Check sheet for the modelled part. Datum: model origin and axes. Units: mm. Face numbers are marked on the shaded views. A direction names the side the tool comes from. Give positions to 0.01 mm unless a question says otherwise; leave off trailing zeros. Write each loop counter-clockwise with the first axis right and the second up, starting at its lowest first coordinate (ties: lowest second). Pieces come first, ordered by that corner, then holes.
from build123d import *

# Parameters (mm, degrees)
F0_R     = 20
F0_R_2   = 12.5
F1_DEPTH = 30
F2_R     = 55
F2_R_2   = 20
F3_DEPTH = 25
F4_R     = 12.5
F5_DEPTH = 25


with BuildPart() as f1:
    # F0 (on Right) → F1 (new body)
    with BuildSketch(Plane.YZ):
        with BuildLine():
            ThreePointArc((22, -76.9155380921), (63.8748776907, -48.1663783152), (80, 0))
            ThreePointArc((80, 0), (63.8748776907, 48.1663783152), (22, 76.9155380921))
            ThreePointArc((22, 76.9155380921), (-80, 0), (22, -76.9155380921))
        make_face()
        Circle(F0_R, mode=Mode.SUBTRACT)
        with BuildLine():
            ThreePointArc((22, 76.9155380921), (63.8748776907, 48.1663783152), (80, 0))
            ThreePointArc((80, 0), (63.8748776907, -48.1663783152), (22, -76.9155380921))
            Line((22, -76.9155380921), (206.875, -24.0361056538))
            ThreePointArc((206.875, -24.0361056538), (175, 0), (206.875, 24.0361056538))
            Line((206.875, 24.0361056538), (22, 76.9155380921))
        make_face()
        with BuildLine():
            ThreePointArc((225, 0), (219.9608992783, 15.0519932235), (206.875, 24.0361056538))
            ThreePointArc((206.875, 24.0361056538), (175, 0), (206.875, -24.0361056538))
            ThreePointArc((206.875, -24.0361056538), (219.9608992783, -15.0519932235), (225, 0))
        make_face()
        with Locations((200, 0)):
            Circle(F0_R_2, mode=Mode.SUBTRACT)
    extrude(amount=F1_DEPTH)

    # F2 (on face) → F3 (join)
    with BuildSketch(Plane.YZ.offset(30)):
        Circle(F2_R)
        Circle(F2_R_2, mode=Mode.SUBTRACT)
    extrude(amount=F3_DEPTH)

    # F4 (on face) → F5 (join)
    with BuildSketch(Plane.YZ.offset(30)):
        with BuildLine():
            ThreePointArc((206.875, -24.0361056538), (219.9608992783, -15.0519932235), (225, 0))
            ThreePointArc((225, 0), (219.9608992783, 15.0519932235), (206.875, 24.0361056538))
            ThreePointArc((206.875, 24.0361056538), (175, 0), (206.875, -24.0361056538))
        make_face()
        with Locations((200, 0)):
            Circle(F4_R, mode=Mode.SUBTRACT)
    extrude(amount=F5_DEPTH)


solid = f1.part
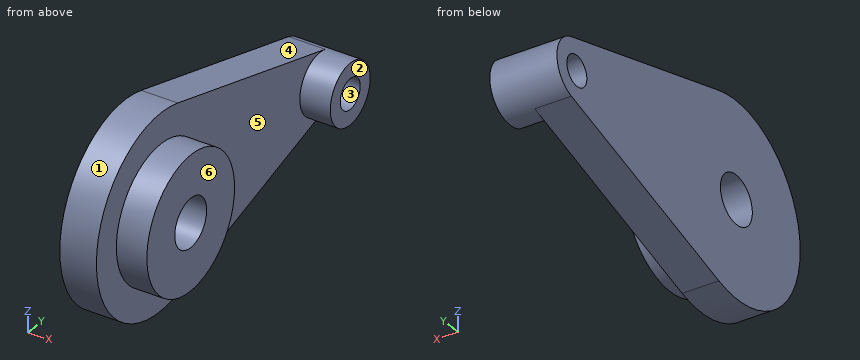
1) Draft check along Z on the marked faces 1, 2, 3 and 4. Enter one of: +Z half, -Z half, draft (parallel to the pull), parting line (faces both ways), or undercut.
2) Gauge pin test, flat ends, axial feed: pin 1 (5 mm diameter, centred on x = 12.5, z = 33.5, fed in from -Y); pin 2 (1 mm diameter, centred on x = 35, y = 47, fed in from -Z); pin 3 (6 mm diameter, centred on x = 42, y = -27.5, fed in from +Z); pin 4 (1.5 mm diameter, centred on y = 78.5, z = -31, fed in from -X). Record the tip position at first contact, or that the pin passes through.
3) Sectioned sample at C-C on x = 12. Record the boundary of the cut face in (y, z) (3 decimals), then the cut area to 3 significant figures.
4) Sectioned sample at A-A on z = 0. Record the boundary of the cut face in (x, y).
5) Scan lines: L1, parallel to Z at x = 32.5, y = 0; L2, parallel to Z at x = 20, y = 0; L3, parallel to X at y = -39, z = -55. Record each from-to range of solid material in increasing order.
6) Sectioned sample at D-D on x = 51. Record the boundary of the cut face in (y, z) (3 decimals), then the cut area to 3 significant figures.
7) Access from +Z, -Z, +X, -X, +Y, -Y to the whole of each face (thin tool, end or side, straight path). Record for the marked faces 5 and 6.
8) Sectioned sample at B-B on y = 0. Record the boundary of the cut face in (x, z).
Answers below:
1. face 1: parting line
1. face 2: draft
1. face 3: undercut
1. face 4: +Z half
2. pin 1: stops at y = -73.75
2. pin 2: stops at z = -29.37
2. pin 3: stops at z = 49.24
2. pin 4: stops at x = 0
3. outline: (22, -76.916) - (206.875, -24.036) arc R25 ccw to (206.875, 24.036) - (22, 76.916) arc R80 ccw (long way) to start; hole circle Ø40 at (0, 0); hole circle Ø25 at (200, 0)
3. area: 31,100 mm2
4. outline: (0, -80) - (30, -80) - (30, -55) - (55, -55) - (55, -20) - (0, -20) - close; (0, 20) - (55, 20) - (55, 55) - (30, 55) - (30, 175) - (55, 175) - (55, 187.5) - (0, 187.5) - close; (0, 212.5) - (55, 212.5) - (55, 225) - (0, 225) - close
5. L1: z = -55 to -20, 20 to 55
5. L2: z = -80 to -20, 20 to 80
5. L3: x = 0 to 30
6. outline: circle Ø110 at (0, 0); circle Ø50 at (200, 0); hole circle Ø40 at (0, 0); hole circle Ø25 at (200, 0)
6. area: 9,720 mm2
7. face 5: +X
7. face 6: +Z, -Z, +X, +Y, -Y
8. outline: (0, -80) - (30, -80) - (30, -55) - (55, -55) - (55, -20) - (0, -20) - close; (0, 20) - (55, 20) - (55, 55) - (30, 55) - (30, 80) - (0, 80) - close
